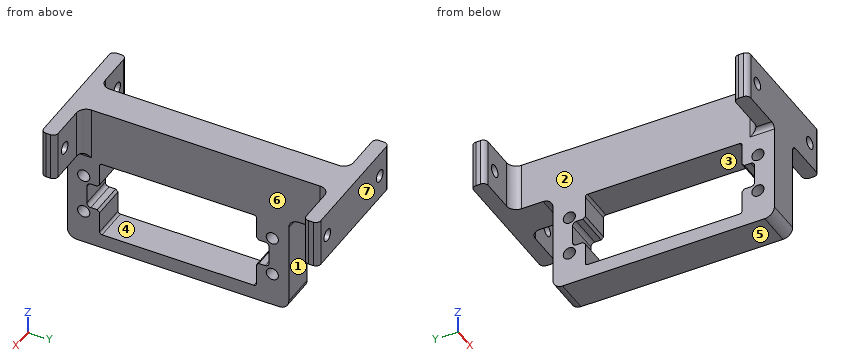
from build123d import *

# Parameters (mm, degrees)
FRAME_MOUNT_DEPTH         = 12.7
SKETCH3_R                 = 1.5875000000000008
SKETCH3_R_2               = 1.5875000000000024
MOUNT_HOLES_DEPTH         = 76.8344213797402
SKETCH4_W                 = 20.574
SKETCH4_H                 = 41.148
SERVO_MOUNT_FEATURE_DEPTH = 8.889999999999999
SKETCH5_R                 = 1.6001999999999992
SKETCH5_R_2               = 1.6001999999999998
SKETCH5_R_3               = 1.6002000000000005
SKETCH5_R_4               = 1.600200000000004
SERVO_MOUNT_HOLES_DEPTH   = 81.41316677012539
FILLET1_R                 = 2.54
FILLET2_R                 = 1.27
FILLET3_R                 = 0.635
FILLET4_R                 = 1.27
SKETCH6_W                 = 6.8580000000000005
SKETCH6_H                 = 3.352800000000009
SKETCH6_H_2               = 3.352800000000002
SERVOWIRE_GAP_DEPTH       = 81.41316677012539
FILLET5_R                 = 1.016
CHAMFER1_SIZE             = 0.635


with BuildPart() as part:
    # Sketch1 → Frame_Mount (new body)
    with BuildSketch(Plane.XY):
        Polygon((17.144999999999985, -4.04e-15), (-17.144999999999985, -4.04e-15), (-17.144999999999985, 3.809999999999992), (-4.444999999999985, 3.809999999999999), (-4.444999999999985, 68.96100000000001), (-17.144999999999985, 68.961), (-17.144999999999985, 72.77099999999999), (17.144999999999985, 72.77099999999999), (17.145000000000014, 68.961), (4.445000000000014, 68.961), (4.445000000000014, 3.809999999999999), (17.145000000000014, 3.8099999999999863), align=None)
    extrude(amount=FRAME_MOUNT_DEPTH)

    # Sketch3 → Mount_Holes (cut, through all)
    with BuildSketch(Plane.XZ):
        with Locations((12.7, 6.35)):
            Circle(SKETCH3_R)
        with Locations((-12.7, 6.35)):
            Circle(SKETCH3_R_2)
    extrude(amount=-MOUNT_HOLES_DEPTH, mode=Mode.SUBTRACT)

    # Sketch4 → Servo_Mount_Feature (add)
    with BuildSketch(Plane(origin=(4.445000000000014, 0, 0), x_dir=(0, 0, -1), z_dir=(1, 3.9e-16, 0))):
        Polygon((7.11e-15, 58.166000000000004), (26.543000000000006, 58.166), (26.543000000000006, -6.94e-15), (6.94e-15, -9.04e-15), align=None)
        with Locations((12.446000000000007, 29.082999999999995)):
            Rectangle(SKETCH4_W, SKETCH4_H, mode=Mode.SUBTRACT)
    extrude(amount=-SERVO_MOUNT_FEATURE_DEPTH)

    # Sketch5 → Servo_Mount_Holes (cut, through all)
    with BuildSketch(Plane(origin=(4.445000000000014, 0, 0), x_dir=(0, 0, -1), z_dir=(1, 3.9e-16, 0))):
        with Locations(Location((7.239000000000005, 53.84799999999999, 0), (0, 0, 90))):
            Circle(SKETCH5_R)
        with Locations((17.653000000000006, 53.84799999999999)):
            Circle(SKETCH5_R_2)
        with Locations(Location((17.653000000000006, 4.318000000000002, 0), (0, 0, 90))):
            Circle(SKETCH5_R_3)
        with Locations((7.239000000000006, 4.317999999999992)):
            Circle(SKETCH5_R_4)
    extrude(amount=-SERVO_MOUNT_HOLES_DEPTH, mode=Mode.SUBTRACT)

    # Fillet1
    fillet1_edges = [part.edges().sort_by_distance(p)[0] for p in [
        (-4.444999999999985, 3.809999999999999, 6.35),
        (-4.444999999999985, 68.96100000000001, 6.35),
        (4.445000000000014, 68.961, 6.35),
        (4.445000000000014, 3.809999999999999, 6.35),
        (-8.88e-15, 58.166000000000004, -7.11e-15),
        (-8.88e-15, 58.166, -26.543000000000006),
        (1.421e-14, -8.69e-15, -26.543000000000006),
    ]]
    fillet(fillet1_edges, radius=FILLET1_R)

    # Fillet2
    fillet2_edges = [part.edges().sort_by_distance(p)[0] for p in [
        (-4.444999999999986, 3.174999999999993, -3.47e-15),
        (4.445000000000013, 3.174999999999993, -3.47e-15),
    ]]
    fillet(fillet2_edges, radius=FILLET2_R)

    # Fillet3
    fillet3_edges = [part.edges().sort_by_distance(p)[0] for p in [
        (-5.33e-15, 49.65699999999999, -2.159000000000006),
        (-5.33e-15, 49.65699999999999, -22.733000000000008),
        (1.066e-14, 8.508999999999993, -22.733000000000008),
        (1.066e-14, 8.508999999999993, -2.159000000000006),
    ]]
    fillet(fillet3_edges, radius=FILLET3_R)

    # Fillet4
    fillet4_edges = [part.edges().sort_by_distance(p)[0] for p in [
        (-17.144999999999985, 3.809999999999992, 6.35),
        (-17.144999999999985, 68.961, 6.35),
        (-17.144999999999985, 72.77099999999999, 6.35),
        (17.144999999999985, 72.77099999999999, 6.35),
        (17.145000000000014, 68.961, 6.35),
        (17.145000000000014, 3.8099999999999863, 6.35),
        (17.144999999999985, -4.04e-15, 6.35),
        (-17.144999999999985, -4.04e-15, 6.35),
    ]]
    fillet(fillet4_edges, radius=FILLET4_R)

    # Sketch6 → ServoWire-Gap (cut, through all)
    with BuildSketch(Plane(origin=(4.445000000000014, 0, 0), x_dir=(0, 0, -1), z_dir=(1, 0, 0))):
        with Locations((12.446000000000007, 51.3334)):
            Rectangle(SKETCH6_W, SKETCH6_H)
        with Locations((12.446000000000007, 6.832599999999994)):
            Rectangle(SKETCH6_W, SKETCH6_H_2)
    extrude(amount=-SERVOWIRE_GAP_DEPTH, mode=Mode.SUBTRACT)

    # Fillet5
    fillet5_edges = [part.edges().sort_by_distance(p)[0] for p in [
        (3.55e-15, 53.009800000000006, -9.017000000000007),
        (3.55e-15, 53.009800000000006, -15.875000000000007),
        (1.332e-14, 5.156199999999993, -15.875000000000007),
        (1.332e-14, 5.156199999999993, -9.017000000000007),
    ]]
    fillet(fillet5_edges, radius=FILLET5_R)

    # Chamfer1
    chamfer1_edges = [part.edges().sort_by_distance(p)[0] for p in [
        (1.243e-14, 8.508999999999995, -9.017000000000007),
        (1.243e-14, 8.508999999999995, -15.875000000000007),
        (4.44e-15, 49.657, -9.017000000000007),
        (4.44e-15, 49.657, -15.875000000000007),
    ]]
    chamfer(chamfer1_edges, length=CHAMFER1_SIZE)


solid = part.part
Here's how the part is built. I have some questions about the finished solid (model axes, mm). Face numbers are marked on the shaded views. A direction names the side the tool comes from. Give positions to 0.01 mm unless a question says otherwise; leave off trailing zeros. Order: outer loops, then holes, each group sorted by start corner. A loop starts at its lowest first (then second) coordinate and runs counter-clockwise, first axis right, second up. Notation, with made-up numbers: (60.5, -23) -> (101.5, -23) arc R31 ccw to (101.5, 13) -> close; hole circle Ø1 at (13.5, 13). An arc over 180 degrees is marked (long way). One line per item, written item: value. Start each with the question number.
1. I need wall thicknesses on probe 1 along Z at (x, y) = (12.7, 71.3); probe 2 along Y at (x, z) = (11, 1); probe 3 along Y at (x, z) = (-2, -12). Which ranges of each line are inside material? Lowest first, please. Write a range as from..to.
2. For the marked faces 1, 2 and 3, which set-ups out of +Z, -Z, +X, -X, +Y, -Y let a thin tool reach every point of the face, with its end or its side?
3. Imagine slicing it at C-C, the plane z = 1. List the corners of the cut face in (x, y) for me (3 decimals).
4. We'd pull the mould along Y, two halves only. Please class the marked faces 4, 5, 6 and 7: released by +Y, released by -Y, zero draft, split by the parting line, or undercut.
5. Imagine slicing it at D-D, the plane x = -13. List the corners of the cut face in (y, z) for me, plus the area to 3 significant figures.
6. Imagine slicing it at B-B, the plane y = 33. List the corners of the cut face in (x, z) for me (3 decimals).
7. Imagine slicing it at A-A, the plane x = 9.5. List the corners of the cut face in (y, z) for me.
8. Will these pins go through, and if not, where does the flat tip stop? pin 1 Ø2.5 at (x, z) = (12.7, 6.35) entering from -Y; pin 2 Ø5 at (y, z) = (56.5, -3) entering from +X (3 decimals); pin 3 Ø3.5 at (x, y) = (-6.5, 68.5) entering from -Z; pin 4 Ø12 at (y, z) = (30.5, -1) entering from -X (3 decimals).
Values follow:
1. probe 1: z = 0..4.76, 7.94..12.7
1. probe 2: y = 0..3.81, 68.96..72.77
1. probe 3: y = 0..5.16, 53.01..58.17
2. face 1: -Z, +X, -X, +Y
2. face 2: -Z, -X
2. face 3: +X, -X
3. outline: (-17.145, 1.27) arc R1.27 ccw to (-15.875, 0) -> (15.875, 0) arc R1.27 ccw to (17.145, 1.27) -> (17.145, 2.54) arc R1.27 ccw to (15.875, 3.81) -> (6.985, 3.81) arc R2.54 cw to (4.445, 6.35) -> (4.445, 66.421) arc R2.54 cw to (6.985, 68.961) -> (15.875, 68.961) arc R1.27 ccw to (17.145, 70.231) -> (17.145, 71.501) arc R1.27 ccw to (15.875, 72.771) -> (-15.875, 72.771) arc R1.27 ccw to (-17.145, 71.501) -> (-17.145, 70.231) arc R1.27 ccw to (-15.875, 68.961) -> (-6.985, 68.961) arc R2.54 cw to (-4.445, 66.421) -> (-4.445, 6.35) arc R2.54 cw to (-6.985, 3.81) -> (-15.875, 3.81) arc R1.27 ccw to (-17.145, 2.54) -> close
4. face 4: undercut
4. face 5: zero draft
4. face 6: undercut
4. face 7: released by +Y
5. outline: (0, 0) -> (3.81, 0) -> (3.81, 4.79) -> (0, 4.79) -> close; (0, 7.91) -> (3.81, 7.91) -> (3.81, 12.7) -> (0, 12.7) -> close; (68.96, 0) -> (72.77, 0) -> (72.77, 4.79) -> (68.96, 4.79) -> close; (68.96, 7.91) -> (72.77, 7.91) -> (72.77, 12.7) -> (68.96, 12.7) -> close
5. area: 73.0 mm2
6. outline: (-4.445, -26.543) -> (4.445, -26.543) -> (4.445, -22.733) -> (-4.445, -22.733) -> close; (-4.445, -2.159) -> (4.445, -2.159) -> (4.445, 12.7) -> (-4.445, 12.7) -> close
7. outline: (0, 0) -> (3.81, 0) -> (3.81, 12.7) -> (0, 12.7) -> close; (68.96, 0) -> (72.77, 0) -> (72.77, 12.7) -> (68.96, 12.7) -> close
8. pin 1: passes through
8. pin 2: stops at x = 4.445
8. pin 3: stops at z = 0
8. pin 4: stops at x = -4.445
